Geometry: final body of the model. Coordinates: model frame, mm. Face numbers are marked on the shaded views. A direction names the side the tool comes from. Round coordinates to 2 decimals unless told otherwise and drop trailing zeros. Loops run counter-clockwise (first coordinate to the right, second up) from the corner with the lowest first, then second, coordinate; pieces in that order, holes last. Notation, with made-up numbers: (75.5, -40) -> (96.5, -40) arc R10 ccw to (96.5, -25) -> close; hole circle Ø11 at (-10.75, -10). An arc over 180 degrees is marked (long way). Answer in a Markdown table with one row per item.
```python
from build123d import *

# Parameters (mm, degrees)
SKETCH1_R           = 7.5
BOSS_EXTRUDE1_DEPTH = 4
SKETCH2_R           = 5
BOSS_EXTRUDE2_DEPTH = 15
SKETCH3_R           = 4
CUT_EXTRUDE1_DEPTH  = 7


with BuildPart() as part:
    # Sketch1 → Boss-Extrude1 (new body)
    with BuildSketch(Plane.XY):
        Circle(SKETCH1_R)
    extrude(amount=BOSS_EXTRUDE1_DEPTH)

    # Sketch2 → Boss-Extrude2 (add)
    with BuildSketch(Plane.XY.offset(4)):
        Circle(SKETCH2_R)
    extrude(amount=BOSS_EXTRUDE2_DEPTH)

    # Sketch3 → Cut-Extrude1 (cut, symmetric)
    with BuildSketch(Plane(origin=(0, 0, 0), x_dir=(1, 0, 0), z_dir=(0, 1, 0))):
        with Locations((0, -13)):
            Circle(SKETCH3_R)
    extrude(amount=CUT_EXTRUDE1_DEPTH, both=True, mode=Mode.SUBTRACT)


solid = part.part
```
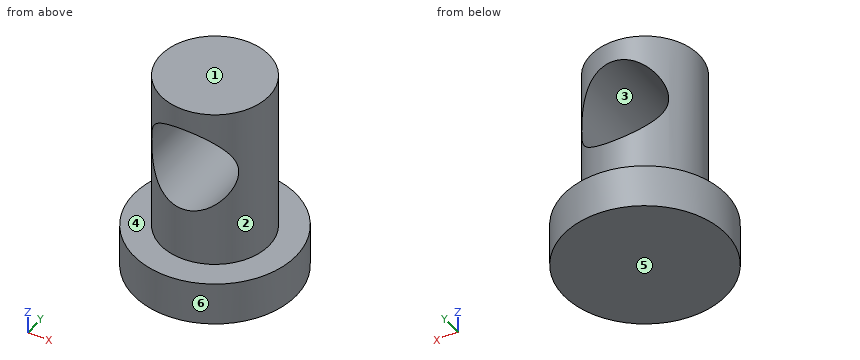
Item 1: Pin query (flat end, axial travel): pin 1 Ø6 at (x, z) = (4, 5) entering from +Y; pin 2 Ø6 at (x, z) = (3.5, 15) entering from +Y; pin 3 Ø2 at (y, z) = (2.5, 13.5) entering from +X; pin 4 Ø7 at (x, z) = (0, 13) entering from -Y. Return the tip coordinate at first contact, or that it passes through.
Answer:
| item | result |
|---|---|
| pin 1 | stops at y = 7.41 |
| pin 2 | stops at y = 4.87 |
| pin 3 | stops at x = 4.77 |
| pin 4 | passes through |
Item 2: Cut plane D-D (y = -3.75). Output: boundary loops of the cut face in (x, z).
Answer:
| item | result |
|---|---|
| outline | (-6.5, 0) -> (6.5, 0) -> (6.5, 4) -> (3.31, 4) -> (3.31, 10.75) arc R4 cw to (-3.31, 10.75) -> (-3.31, 4) -> (-6.5, 4) -> close; (-3.31, 15.25) arc R4 cw to (3.31, 15.25) -> (3.31, 19) -> (-3.31, 19) -> close |
Item 3: Cut plane C-C (z = 13). Output: boundary loops of the cut face in (x, y).
Answer:
| item | result |
|---|---|
| outline | (-4, -3) -> (-4, 3) arc R5 ccw to start; (4, -3) arc R5 ccw to (4, 3) -> close |
Item 4: Cut plane A-A (x = 0). Output: boundary loops of the cut face in (y, z), then the cut area to 3 significant figures.
Answer:
| item | result |
|---|---|
| outline | (-7.5, 0) -> (7.5, 0) -> (7.5, 4) -> (5, 4) -> (5, 9) -> (-5, 9) -> (-5, 4) -> (-7.5, 4) -> close; (-5, 17) -> (5, 17) -> (5, 19) -> (-5, 19) -> close |
| area | 130 mm² |
Item 5: Draft query along Z for the marked faces 3, 4, 5 and 6. Return one class per face: pulls with the +Z half, pulls with the -Z half, needs draft (parallel to the pull), parting line crosses it, or undercut.
Answer:
| item | result |
|---|---|
| face 3 | undercut |
| face 4 | pulls with the +Z half |
| face 5 | pulls with the -Z half |
| face 6 | needs draft |
Item 6: Line query: probe 1 along Z at (x, y) = (0, 0.75); probe 2 along Z at (x, y) = (-5.25, 3.5); probe 3 along X at (y, z) = (2.75, 15). Output: solid intervals per line, ascending. Write a range as [from, to].
Answer:
| item | result |
|---|---|
| probe 1 | z = [0, 9], [17, 19] |
| probe 2 | z = [0, 4] |
| probe 3 | x = [-4.18, -3.46], [3.46, 4.18] |
Item 7: Cut plane B-B (y = 0). Output: boundary loops of the cut face in (x, z).
Answer:
| item | result |
|---|---|
| outline | (-7.5, 0) -> (7.5, 0) -> (7.5, 4) -> (5, 4) -> (5, 19) -> (-5, 19) -> (-5, 4) -> (-7.5, 4) -> close; hole circle Ø8 at (0, 13) |
Item 8: Reachability of the marked faces 1 and 2 from +Z, -Z, +X, -X, +Y, -Y: full face, straight path, thin tool, end or side. Return the list, or none.
Answer:
| item | result |
|---|---|
| face 1 | +Z, +X, -X, +Y, -Y |
| face 2 | +Z |
